For this review, take the finished solid that the model builds, in its own axes (mm). A direction names the side the tool comes from. Give positions to 0.01 mm unless a question says otherwise; leave off trailing zeros. Order: outer loops, then holes, each group sorted by start corner. A loop starts at its lowest first (then second) coordinate and runs counter-clockwise, first axis right, second up. Notation, with made-up numbers: (61, -35.75) -> (71, -35.75) arc R24 ccw to (71, 0.25) -> close; hole circle Ø9 at (83, 24). An arc over 180 degrees is marked (long way). One line per item, written item: value. Start each with the question number.
from build123d import *

# Parameters (mm, degrees)
F1_DEPTH = 25.4
F3_DEPTH = 25.4
F4_R     = 6.591123
F4_R_2   = 6.739643
F5_DEPTH = 25.4
F7_DEPTH = 25.4
F8_R     = 5.08
F9_R     = 5.08


with BuildPart() as f1:
    # F0 (on Front) → F1 (new body)
    with BuildSketch(Plane.XZ):
        Polygon((12.7, 44.45), (0, 44.45), (0, 0), (63.5, 0), (63.5, 12.7), (12.7, 12.7), align=None)
    extrude(amount=F1_DEPTH)

    # F2 (on face) → F3 (cut)
    with BuildSketch(Plane.XY.offset(12.7)):
        with BuildLine():
            ThreePointArc((63.5, -14.510555), (59.986844, -21.676886), (52.927312, -25.4))
            Line((52.927312, -25.4), (63.5, -25.4))
            Line((63.5, -25.4), (63.5, -14.510555))
        make_face()
        with BuildLine():
            ThreePointArc((52.927312, 0), (59.986844, -3.723114), (63.5, -10.889445))
            Line((63.5, -10.889445), (63.5, 0))
            Line((63.5, 0), (52.927312, 0))
        make_face()
    extrude(amount=-F3_DEPTH, mode=Mode.SUBTRACT)

    # F4 (on face) → F5 (cut)
    with BuildSketch(Plane.XY.offset(12.7)):
        with Locations((26.618414, -12.7)):
            Circle(F4_R)
        with Locations((47.665533, -12.7)):
            Circle(F4_R_2)
    extrude(amount=-F5_DEPTH, mode=Mode.SUBTRACT)

    # F6 (on face) → F7 (cut)
    with BuildSketch(Plane.YZ.offset(12.7)):
        with BuildLine():
            ThreePointArc((-19.05, 31.75), (-12.7, 25.4), (-6.35, 31.75))
            Line((-6.35, 31.75), (-6.35, 44.45))
            Line((-6.35, 44.45), (-19.05, 44.45))
            Line((-19.05, 44.45), (-19.05, 31.75))
        make_face()
    extrude(amount=-F7_DEPTH, mode=Mode.SUBTRACT)

    # F8
    f8_edges = [f1.edges().sort_by_distance(p)[0] for p in [
        (6.35, -25.4, 44.45),
    ]]
    fillet(f8_edges, radius=F8_R)

    # F9
    f9_edges = [f1.edges().sort_by_distance(p)[0] for p in [
        (6.35, 0, 44.45),
    ]]
    fillet(f9_edges, radius=F9_R)


solid = f1.part
Q1. Take a section at A-A (z = 37). State the section outline as (x, y) points.
Q2. For line 1 along X through (y, z) = (-16.5, 7); line 2 along Z through (x, y) = (8, -4.75); line 3 along Z through (x, y) = (54, -18.75), list the stretches that pass through material, from the lowest coordinate up.
Q3. Take a section at B-B (y = -7.5). State the section outline as (x, z) points, and give its area (3 significant figures).
Q4. Take a section at C-C (x = 43). State the section outline as (y, z) points, and give its area (3 significant figures).
Q5. Mouldability with a two-part tool opening along Y and no side actions: class faces 1 (the cylindrical face through (6.4, -12.8, 25.4)), 2 (the flat face through (20, -25.4, 11)), 3 (the flat face through (0, -13, 18)) as pulls with the +Y half, pulls with the -Y half, needs draft (parallel to the pull), parting line crosses it, or undercut.
Q6. For pin 1 Ø1 at (y, z) = (-13.5, 22.5) entering from -X; pin 2 Ø4 at (x, y) = (18.5, -18) entering from +Z; pin 3 Ø2 at (y, z) = (-8.5, 17) entering from +X, all flat-tipped, find the tip position at first contact; note any pin that passes through.
Q7. Take a section at D-D (x = 4.5). State the section outline as (y, z) points, and give its area (3 significant figures).
Q8. For faces 4 (the flat face through (38, -13, 12.7)), 5 (the flat face through (6, -6.35, 38)), 6 (the flat face through (63.5, -13, 6)), list the 3-axis set-ups (+Z, -Z, +X, -X, +Y, -Y) from which the entire face can be reached by the end or side of a thin tool; tool diameter is ignored.
Answers below:
1. outline: (0, -25.4) -> (12.7, -25.4) -> (12.7, -19.05) -> (0, -19.05) -> close; (0, -6.35) -> (12.7, -6.35) -> (12.7, 0) -> (0, 0) -> close
2. line 1: x = 0 to 21.23, 32 to 42.1, 53.23 to 63.05
2. line 2: z = 0 to 44.44
2. line 3: z = 0 to 12.7
3. outline: (0, 0) -> (22.57, 0) -> (22.57, 12.7) -> (12.7, 12.7) -> (12.7, 28.11) -> (0, 28.11) -> close; (30.67, 0) -> (43.38, 0) -> (43.38, 12.7) -> (30.67, 12.7) -> close; (51.95, 0) -> (62.53, 0) -> (62.53, 12.7) -> (51.95, 12.7) -> close
3. area: 778 mm²
4. outline: (-25.4, 0) -> (-17.56, 0) -> (-17.56, 12.7) -> (-25.4, 12.7) -> close; (-7.84, 0) -> (0, 0) -> (0, 12.7) -> (-7.84, 12.7) -> close
4. area: 199 mm²
5. face 1: undercut
5. face 2: pulls with the -Y half
5. face 3: needs draft
6. pin 1: stops at x = 0
6. pin 2: stops at z = 12.7
6. pin 3: stops at x = 12.7
7. outline: (-25.4, 0) -> (0, 0) -> (0, 39.37) arc R5.08 ccw to (-5.08, 44.45) -> (-6.35, 44.45) -> (-6.35, 31.75) arc R6.35 cw to (-19.05, 31.75) -> (-19.05, 44.45) -> (-20.32, 44.45) arc R5.08 ccw to (-25.4, 39.37) -> close
7. area: 893 mm²
8. face 4: +Z, +X, +Y, -Y
8. face 5: +Z, +X, -X
8. face 6: +Z, -Z, +X, +Y, -Y
